Autodesk Fusion 360 part; units mm, degrees
sketch "Sketch: plate" plane through (0, 0, 0) normal (0, 0, 1) x (1, 0, 0)
  line L0 (-111, 0.4) -> (111, 0.4)
  line L1 (111, 0.4) -> (111, 132.95)
  line L2 (111, 132.95) -> (-111, 132.95)
  line L3 (-111, 132.95) -> (-111, 0.4)
extrude "Plate" add sketch "Sketch: plate" along normal blind 4
sketch "Sketch: duct walls" plane through (0, 0, 0) normal (0, 0, 1) x (1, 0, 0)
  line L0 (-96.72, 2.1) -> (96.72, 2.1)
  line L1 (96.72, 2.1) -> (96.72, 4.3)
  line L2 (96.72, 4.3) -> (-96.72, 4.3)
  line L3 (-96.72, 4.3) -> (-96.72, 2.1)
  line L4 (-96.72, 129.05) -> (96.72, 129.05)
  line L5 (96.72, 129.05) -> (96.72, 131.25)
  line L6 (96.72, 131.25) -> (-96.72, 131.25)
  line L7 (-96.72, 131.25) -> (-96.72, 129.05)
extrude "Duct walls" add sketch "Sketch: duct walls" against normal blind 72
sketch "Sketch: openings and holes" plane through (0, 0, 0) normal (0, 0, 1) x (1, 0, 0)
  circle A0 centre (0, 66.675) radius 57
  circle A1 centre (-52.5, 14.175) radius 2.25
  circle A2 centre (-52.5, 119.175) radius 2.25
  circle A3 centre (52.5, 14.175) radius 2.25
  circle A4 centre (52.5, 119.175) radius 2.25
  circle A5 centre (-102.82, 15) radius 1.7
  circle A6 centre (-102.82, 29.45) radius 1.7
  circle A7 centre (-102.82, 59.45) radius 1.7
  circle A8 centre (-102.82, 73.9) radius 1.7
  circle A9 centre (-102.82, 103.9) radius 1.7
  circle A10 centre (-102.82, 118.35) radius 1.7
  circle A11 centre (102.82, 15) radius 1.7
  circle A12 centre (102.82, 29.45) radius 1.7
  circle A13 centre (102.82, 59.45) radius 1.7
  circle A14 centre (102.82, 73.9) radius 1.7
  circle A15 centre (102.82, 103.9) radius 1.7
  circle A16 centre (102.82, 118.35) radius 1.7
extrude "Openings and holes" cut sketch "Sketch: openings and holes" along normal blind 4
sketch "Sketch: tie slots" plane through (0, 0, 0) normal (0, 0, 1) x (1, 0, 0)
  line L0 (70.75, 59.425) -> (73.25, 59.425)
  line L1 (73.25, 59.425) -> (73.25, 64.425)
  line L2 (73.25, 64.425) -> (70.75, 64.425)
  line L3 (70.75, 64.425) -> (70.75, 59.425)
  line L4 (70.75, 68.925) -> (73.25, 68.925)
  line L5 (73.25, 68.925) -> (73.25, 73.925)
  line L6 (73.25, 73.925) -> (70.75, 73.925)
  line L7 (70.75, 73.925) -> (70.75, 68.925)
  line L8 (90.75, 59.425) -> (93.25, 59.425)
  line L9 (93.25, 59.425) -> (93.25, 64.425)
  line L10 (93.25, 64.425) -> (90.75, 64.425)
  line L11 (90.75, 64.425) -> (90.75, 59.425)
  line L12 (90.75, 68.925) -> (93.25, 68.925)
  line L13 (93.25, 68.925) -> (93.25, 73.925)
  line L14 (93.25, 73.925) -> (90.75, 73.925)
  line L15 (90.75, 73.925) -> (90.75, 68.925)
extrude "Tie slots" cut sketch "Sketch: tie slots" along normal blind 4
ref_plane "WorkPlane1" through (0, 0, 4) normal (0, 0, 1) x (1, 0, 0)
sketch "Sketch: head counterbores" plane through (0, 0, 4) normal (0, 0, 1) x (1, 0, 0)
  circle A0 centre (-102.82, 15) radius 3.25
  circle A1 centre (-102.82, 29.45) radius 3.25
  circle A2 centre (-102.82, 59.45) radius 3.25
  circle A3 centre (-102.82, 73.9) radius 3.25
  circle A4 centre (-102.82, 103.9) radius 3.25
  circle A5 centre (-102.82, 118.35) radius 3.25
  circle A6 centre (102.82, 15) radius 3.25
  circle A7 centre (102.82, 29.45) radius 3.25
  circle A8 centre (102.82, 59.45) radius 3.25
  circle A9 centre (102.82, 73.9) radius 3.25
  circle A10 centre (102.82, 103.9) radius 3.25
  circle A11 centre (102.82, 118.35) radius 3.25
extrude "Head counterbores" cut sketch "Sketch: head counterbores" against normal blind 2
chamfer "Inlet chamfer" distance 3 angle 45 1 edges at (-53.1427, 46.0629, 0)
The model under review builds one solid part; all positions refer to its coordinate system, in mm. A direction names the side the tool comes from. Round coordinates to 2 decimals unless told otherwise and drop trailing zeros. Write each loop counter-clockwise with the first axis right and the second up, starting at its lowest first coordinate (ties: lowest second). Pieces come first, ordered by that corner, then holes. Notation, with made-up numbers: (13.25, 71) -> (54.25, 71) arc R20 ccw to (54.25, 90) -> close; hole circle Ø11 at (-6, -8.5). An arc over 180 degrees is marked (long way). Answer as a JSON object with one key per item and string values.
1. We need section A-A on x = 0. State the section outline as (y, z) points (3 decimals), and give its area (3 significant figures).
Results found:
{"outline": "(0.4, 0) -> (2.1, 0) -> (2.1, -72) -> (4.3, -72) -> (4.3, 0) -> (6.675, 0) -> (9.675, 3) -> (9.675, 4) -> (0.4, 4) -> close; (123.675, 3) -> (126.675, 0) -> (129.05, 0) -> (129.05, -72) -> (131.25, -72) -> (131.25, 0) -> (132.95, 0) -> (132.95, 4) -> (123.675, 4) -> close", "area": "382 mm^2"}
2. Clearance check with flat-ended pins moving along their axes: pin 1 (2 mm diameter, centred on x = 102.5, y = 16, fed in from +Z); pin 2 (5.5 mm diameter, centred on x = -102.82, y = 29.45, fed in from -Z); pin 3 (2.5 mm diameter, centred on y = 130, z = -22.5, fed in from -X). State where each tip first meets the part, or that it passes through.
Results found:
{"pin 1": "stops at z = 2", "pin 2": "stops at z = 0", "pin 3": "stops at x = -96.72"}
3. Machinability: for faces 1 (the face through (-1, 129.05, -35)), 2 (the face through (105.92, 15.98, 3.01)), 3 (the face through (-12.36, 122.32, 3.49)), which of the approach directions +Z, -Z, +X, -X, +Y, -Y give a long, thin tool a straight path to every point of the face, cutting with its end or side? Answer none if there is none.
Results found:
{"face 1": "-Z, +X, -X", "face 2": "+Z", "face 3": "+Z, -Z"}
4. We need section C-C on x = -63. State the section outline as (y, z) points, and give its area (3 significant figures).
Results found:
{"outline": "(0.4, 0) -> (2.1, 0) -> (2.1, -72) -> (4.3, -72) -> (4.3, 0) -> (129.05, 0) -> (129.05, -72) -> (131.25, -72) -> (131.25, 0) -> (132.95, 0) -> (132.95, 4) -> (0.4, 4) -> close", "area": "847 mm^2"}
5. We need section B-B on z = -4. State the section outline as (x, y) points.
Results found:
{"outline": "(-96.72, 2.1) -> (96.72, 2.1) -> (96.72, 4.3) -> (-96.72, 4.3) -> close; (-96.72, 129.05) -> (96.72, 129.05) -> (96.72, 131.25) -> (-96.72, 131.25) -> close"}
6. To check wall thickness, follow line 1 along X through (y, z) = (15, 0.9); line 2 along Y through (x, z) = (0, 3.5) (3 decimals); line 3 along Y through (x, z) = (52, 1). State the ranges of each line that lie inside material, in increasing order.
Results found:
{"line 1": "x = -111 to -104.52, -101.12 to -54.59, -50.41 to -28.68, 28.68 to 50.41, 54.59 to 101.12, 104.52 to 111", "line 2": "y = 0.4 to 9.675, 123.675 to 132.95", "line 3": "y = 0.4 to 11.98, 16.37 to 38.8, 94.55 to 116.98, 121.37 to 132.95"}
